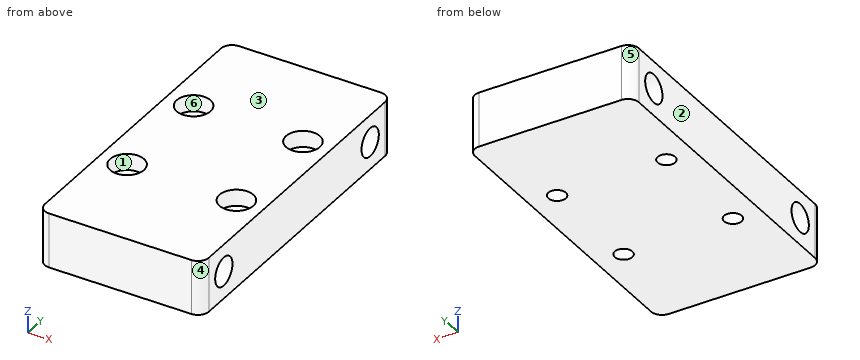
Autodesk Inventor part; units mm, degrees
ref_plane "YZ Plane" through (0, 0, 0) normal (1, 0, 0) x (0, 1, 0)
ref_plane "XZ Plane" through (0, 0, 0) normal (0, 1, 0) x (-1, 0, 0)
ref_plane "XY Plane" through (0, 0, 0) normal (0, 0, 1) x (1, 0, 0)
sketch "Sketch1" plane through (0, 0, 0) normal (0, 0, 1) x (1, 0, 0)
  line L0 (-15, 28.5) -> (15, 28.5)
  line L1 (15, 28.5) -> (15, -28.5)
  line L2 (15, -28.5) -> (-15, -28.5)
  line L3 (-15, -28.5) -> (-15, 28.5)
  line L4 (-10, 10) -> (10, 10) construction
  line L5 (10, 10) -> (10, -10) construction
  line L6 (10, -10) -> (-10, -10) construction
  line L7 (-10, -10) -> (-10, 10) construction
  point P0 (0, 0)
  point P1 (0, 10)
  point P2 (0, 28.5)
  point P3 (10, 0)
  point P4 (15, 0)
  dimension "d0" = 20
  dimension "d1" = 30
  dimension "d2" = 57
extrude "Extrusion1" add sketch "Sketch1" against normal blind 10
hole "Hole1" at (-10, 10, 0) at (10, 10, 0) at (10, -10, 0) at (-10, -10, 0) direction (0, 0, -1) diameter 3.2 end through all counterbore diameter 6.2 counterbore depth 3
sketch "Sketch2" plane through (15, -28.5, 0) normal (1, 0, 0) x (0, 0, -1)
  line L0 (0, 0) -> (0, 57)
  line L1 (0, 0) -> (10, 0)
  line L2 (10, 57) -> (10, 0)
  line L3 (0, 57) -> (10, 57)
  point P0 (0, 28.5)
  point P1 (5, 50.5)
  point P2 (5, 6.5)
  point P3 (5, 57)
  dimension "d12" = 6.5
  dimension "d13" = 6.5
  dimension "d14" = 44
hole "Hole2" at (15, 22, -5) at (15, -22, -5) direction (-1, 0, 0) diameter 5.2 end through all
fillet "Fillet1" radius 2 4 edges at (15, 28.5, -5) (-15, 28.5, -5) (-15, -28.5, -5) (15, -28.5, -5)
properties part number "Adapter Mount"
For this review, take the finished solid that the model builds, in its own axes (mm). Face numbers are marked on the shaded views. A direction names the side the tool comes from. Coordinates: 2 decimals unless noted, no trailing zeros. Loops run counter-clockwise (first coordinate to the right, second up) from the corner with the lowest first, then second, coordinate; pieces in that order, holes last. Notation, with made-up numbers: (10, 66.25) - (53, 66.25) arc R28 ccw to (53, 89.25) - close; hole circle Ø10 at (-37.75, -31). An arc over 180 degrees is marked (long way). Use a Markdown table: item, result. Add a question column.
Item 1: Insertion check: pin 1 Ø3.5 at (x, y) = (10, -10) entering from +Z. The pin has a flat end and moves straight along its axis. Give the tip position at first contact, or say it passes through.
Item 2: Mouldability with a two-part tool opening along Y and no side actions: class the marked faces 3, 4, 5 and 6 as pulls with the +Y half, pulls with the -Y half, needs draft (parallel to the pull), parting line crosses it, or undercut.
Item 3: For line 1 (X direction, y = -10, z = -6); line 2 (Y direction, x = -5, z = -5); line 3 (X direction, y = 10, z = -1.75), list the stretches that pass through material, from the lowest coordinate up.
Item 4: We need section C-C (x = -10). Give the boundary of the cut face in (y, z), and give its area (3 significant figures).
Item 5: Tool access review of the marked faces 1 and 2: name each direction out of +Z, -Z, +X, -X, +Y, -Y from which nothing blocks a thin tool from reaching the whole face with its end or side.
Item 6: We need section A-A (z = -5). Give the boundary of the cut face in (x, y), and give its area (3 significant figures).
Item 7: We need section B-B (y = -10). Give the boundary of the cut face in (x, z).
Item 8: We need section D-D (y = 23). Give the boundary of the cut face in (x, z).
Results list:
| question | item | result |
|---|---|---|
| 1 | pin 1 | stops at z = -3 |
| 2 | face 3 | needs draft |
| 2 | face 4 | pulls with the -Y half |
| 2 | face 5 | pulls with the +Y half |
| 2 | face 6 | undercut |
| 3 | line 1 | x = -15 to -11.6, -8.4 to 8.4, 11.6 to 15 |
| 3 | line 2 | y = -28.5 to -24.6, -19.4 to 19.4, 24.6 to 28.5 |
| 3 | line 3 | x = -15 to -13.1, -6.9 to 6.9, 13.1 to 15 |
| 4 | outline | (-28.5, -10) - (-11.6, -10) - (-11.6, -3) - (-13.1, -3) - (-13.1, 0) - (-28.5, 0) - close; (-8.4, -10) - (8.4, -10) - (8.4, -3) - (6.9, -3) - (6.9, 0) - (-6.9, 0) - (-6.9, -3) - (-8.4, -3) - close; (11.6, -10) - (28.5, -10) - (28.5, 0) - (13.1, 0) - (13.1, -3) - (11.6, -3) - close; hole circle Ø5.2 at (-22, -5); hole circle Ø5.2 at (22, -5) |
| 4 | area | 446 mm^2 |
| 5 | face 1 | +Z |
| 5 | face 2 | +Z, -Z, -X, +Y, -Y |
| 6 | outline | (-15, -26.5) arc R2 ccw to (-13, -28.5) - (13, -28.5) arc R2 ccw to (15, -26.5) - (15, -24.6) - (-15, -24.6) - close; (-15, -19.4) - (15, -19.4) - (15, 19.4) - (-15, 19.4) - close; (-15, 24.6) - (15, 24.6) - (15, 26.5) arc R2 ccw to (13, 28.5) - (-13, 28.5) arc R2 ccw to (-15, 26.5) - close; hole circle Ø3.2 at (-10, -10); hole circle Ø3.2 at (-10, 10); hole circle Ø3.2 at (10, -10); hole circle Ø3.2 at (10, 10) |
| 6 | area | 1,360 mm^2 |
| 7 | outline | (-15, -10) - (-11.6, -10) - (-11.6, -3) - (-13.1, -3) - (-13.1, 0) - (-15, 0) - close; (-8.4, -10) - (8.4, -10) - (8.4, -3) - (6.9, -3) - (6.9, 0) - (-6.9, 0) - (-6.9, -3) - (-8.4, -3) - close; (11.6, -10) - (15, -10) - (15, 0) - (13.1, 0) - (13.1, -3) - (11.6, -3) - close |
| 8 | outline | (-15, -10) - (15, -10) - (15, -7.4) - (-15, -7.4) - close; (-15, -2.6) - (15, -2.6) - (15, 0) - (-15, 0) - close |
